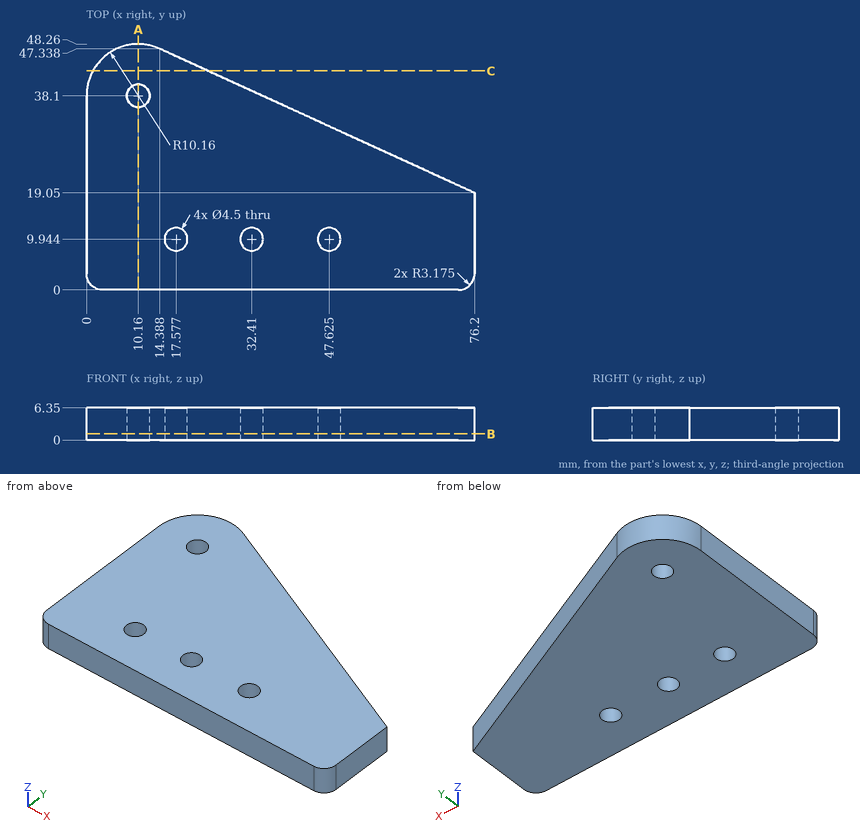
Input: dimensioned drawing with shaded views. Units: mm. Origin: part minimum x, y, z. Coordinates: 2 decimals unless noted, no trailing zeros. Write each loop counter-clockwise with the first axis right and the second up, starting at its lowest first coordinate (ties: lowest second). Pieces come first, ordered by that corner, then holes. Notation, with made-up numbers: M -26.5,28 L 4.5,28 A18 cw 4.5,60 Z; hole C 3.25,33.25 d8. An arc over 180 degrees is marked long. Answer as a JSON object with one key per item and string values. Group by question number.
(1) Section A-A on x = 10.16. Output: boundary loops of the cut face in (y, z), plus the area to 3 significant figures.
(2) Section C-C on y = 43. Output: boundary loops of the cut face in (x, z), plus the area to 3 significant figures.
(3) Ray query, line 1 along Y through (x, z) = (10.16, 3); line 2 along X through (y, z) = (12, 4.5) (1 decimal); line 3 along Y through (x, z) = (17, 6) (1 decimal). Return the intervals inside material, ascending. Write a range as [from, to].
(4) Section B-B on z = 1.25. Give the number of separate pieces and of enclosed holes in the cut face, plus the area to 4 significant figures.
(5) Contact query for a flat-ended pin moving along its axis: P1, Ø1, axis at x = 40, z = 2.5, coming from the +Y side (1 decimal). Output: stop coordinate, or through.
Result set:
{
 "1": {"outline": "M 0,0 L 35.85,0 L 35.85,6.35 L 0,6.35 Z; M 40.35,0 L 48.26,0 L 48.26,6.35 L 40.35,6.35 Z", "area": "278 mm2"},
 "2": {"outline": "M 1.26,0 L 23.87,0 L 23.87,6.35 L 1.26,6.35 Z", "area": "144 mm2"},
 "3": {"line 1": "y = [0, 35.85], [40.35, 48.26]", "line 2": "x = [0, 16.7], [18.5, 31.5], [33.3, 46.7], [48.5, 76.2]", "line 3": "y = [0, 7.8], [12.1, 46.1]"},
 "4": {"separate pieces": "1", "enclosed holes": "4", "area": "2,655 mm2"},
 "5": {"P1": "stops at y = 35.8"}
}
